from build123d import *

# Parameters (mm, degrees)
SKETCH1_W               = 20
SKETCH1_H               = 13
BOSS_EXTRUDE1_DEPTH     = 3
SKETCH2_R               = 1.8
CUT_EXTRUDE1_DEPTH      = 1
CUT_EXTRUDE1_DEPTH_BACK = 4


with BuildPart() as part:
    # Sketch1 → Boss-Extrude1 (new body)
    with BuildSketch(Plane(origin=(0, 0, 0), x_dir=(1, 0, 0), z_dir=(0, 1, 0))):
        with Locations((10, 6.5)):
            Rectangle(SKETCH1_W, SKETCH1_H)
    extrude(amount=BOSS_EXTRUDE1_DEPTH)

    # Sketch2 → Cut-Extrude1 (cut, two sides)
    with BuildSketch(Plane(origin=(0, 3, 0), x_dir=(1, 0, 0), z_dir=(0, 1, 0))) as cut_extrude1_sk:
        with Locations((3.3, 6.5)):
            Circle(SKETCH2_R)
        with Locations((16.7, 6.5)):
            Circle(SKETCH2_R)
    extrude(amount=CUT_EXTRUDE1_DEPTH, mode=Mode.SUBTRACT)
    extrude(cut_extrude1_sk.sketch, amount=-CUT_EXTRUDE1_DEPTH_BACK, mode=Mode.SUBTRACT)


solid = part.part
The model under review builds one solid part; all positions refer to its coordinate system, in mm. Round coordinates to 2 decimals unless told otherwise and drop trailing zeros. Write each loop counter-clockwise with the first axis right and the second up, starting at its lowest first coordinate (ties: lowest second). Pieces come first, ordered by that corner, then holes. Notation, with made-up numbers: M 86,19 L 111,19 A15 ccw 111,42 Z; hole C 17.25,33 d11. An arc over 180 degrees is marked long. Answer as CSV lines item,"result". Start each with the question number.
Q1. Consider section D-D, the plane x = 2.75. Give the boundary of the cut face in (y, z).
Q2. Consider section C-C, the plane y = 2.6. Give the boundary of the cut face in (x, z), then the cut area to 3 significant figures.
Q3. Consider section B-B, the plane x = 16.7. Give the boundary of the cut face in (y, z), then the cut area to 3 significant figures.
Q4. The part is to be moulded in two halves that separate along X. For faces 1 (the face through (0, 1, -6)), 2 (the face through (20, 1, -6)), 3 (the face through (14.9, 1.52, -6.58)), say which applies: +X half, -X half, draft (parallel to the pull), parting line (faces both ways), or undercut.
Q5. Wall thickness on line 1 along X through (y, z) = (1.5, -6.5); line 2 along Z through (x, y) = (3.3, 1.8); line 3 along Z through (x, y) = (3.75, 1.8): over which ranges is each line inside the solid? List them lowest first.
Q6. Consider section A-A, the plane z = -6.5. Give the boundary of the cut face in (x, y), then the cut area to 3 significant figures.
Q7. Clearance check with a flat-ended pin moving along its axis: P1, Ø3, axis at x = 3.3, z = -6.5, coming from the +Y side. State where the tip first meets the part, or that it passes through.
Result set:
1,outline,"M 0,-13 L 3,-13 L 3,-8.21 L 0,-8.21 Z; M 0,-4.79 L 3,-4.79 L 3,0 L 0,0 Z"
2,outline,"M 0,-13 L 20,-13 L 20,0 L 0,0 Z; hole C 3.3,-6.5 d3.6; hole C 16.7,-6.5 d3.6"
2,area,"240 mm²"
3,outline,"M 0,-13 L 3,-13 L 3,-8.3 L 0,-8.3 Z; M 0,-4.7 L 3,-4.7 L 3,0 L 0,0 Z"
3,area,"28.2 mm²"
4,face 1,"-X half"
4,face 2,"+X half"
4,face 3,"undercut"
5,line 1,"x = 0 to 1.5, 5.1 to 14.9, 18.5 to 20"
5,line 2,"z = -13 to -8.3, -4.7 to 0"
5,line 3,"z = -13 to -8.24, -4.76 to 0"
6,outline,"M 0,0 L 1.5,0 L 1.5,3 L 0,3 Z; M 5.1,0 L 14.9,0 L 14.9,3 L 5.1,3 Z; M 18.5,0 L 20,0 L 20,3 L 18.5,3 Z"
6,area,"38.4 mm²"
7,P1,"passes through"
